Here's how the part is built. I have some questions about the finished solid (model axes, mm). A direction names the side the tool comes from. Coordinates: 2 decimals unless noted, no trailing zeros. Order: outer loops, then holes, each group sorted by start corner. A loop starts at its lowest first (then second) coordinate and runs counter-clockwise, first axis right, second up. Notation, with made-up numbers: M 15.5,56 L 24.5,56 A25 cw 24.5,75 Z; hole C -15.5,7.5 d2. An arc over 180 degrees is marked long. Answer as CSV lines item,"result". Start each with the question number.
Autodesk Inventor part; units mm, degrees
ref_plane "Start plane" through (0, 0, 0) normal (0, 0, 1) x (1, 0, 0)
ref_plane "End plane" through (0, 0, 1323.975) normal (0, 0, 1) x (1, 0, 0)
ref_plane "YZ Plane" through (0, 0, 0) normal (1, 0, 0) x (0, 1, 0)
ref_plane "Start plane" through (0, 0, 0) normal (0, 0, 1) x (1, 0, 0)
ref_plane "End plane" through (0, 0, 1323.975) normal (0, 0, 1) x (1, 0, 0)
sketch "Sketch" plane through (0, 0, 0) normal (0, 0, 1) x (1, 0, 0)
  line L0 (0, 76.2) -> (0, 0)
  line L1 (0, 0) -> (50.8, 0)
  line L2 (50.8, 0) -> (50.8, 2.7625)
  line L3 (48.8, 4.7625) -> (12.6365, 4.7625)
  line L4 (4.7625, 12.6365) -> (4.7625, 74.2)
  line L5 (2.7625, 76.2) -> (0, 76.2)
  line L6 (-7.0414, 0) -> (21.5385, 0) construction
  line L7 (0, -8.0414) -> (0, 34.5385) construction
  arc A0 (4.7625, 12.6365) -> (12.6365, 4.7625) centre (12.6365, 12.6365) ccw
  arc A1 (50.8, 2.7625) -> (48.8, 4.7625) centre (48.8, 2.7625) ccw
  arc A2 (4.7625, 74.2) -> (2.7625, 76.2) centre (2.7625, 74.2) ccw
  line L8 (0, 93.5453) -> (0, -24.9725) construction
  line L9 (-18.6925, 0) -> (62.8653, 0) construction
  point P0 (50.8, 4.7625)
  point P1 (4.7625, 4.7625)
  point P2 (4.7625, 76.2)
  dimension "d12" = 4.7625
  dimension "d13" = 76.2
  dimension "d14" = 50.8
  dimension "d15" = 0
  dimension "d16" = 4.7625
  dimension "d17" = 0
  dimension "d18" = 7.874
  dimension "d19" = 2
extrude "Body" add sketch "Sketch" along normal up to surface (1323.975 mm away) from surface at 0
equation "\"d12\" = G_T"
equation "\"d13\" = G_H"
equation "\"d14\" = G_W"
equation "\"d16\" = G_T"
equation "\"d18\" = G_IR"
equation "\"d4\" = G_L"
equation "\"G_W\" = 50.8"
equation "\"G_H\" = 76.2"
equation "\"G_T\" = 4.7625"
equation "\"G_ER\" = 4.064"
equation "\"G_IR\" = 7.874"
equation "\"G_L\" = B_L + G_OFFSET_START + G_OFFSET_END"
equation "\"ex\" = 0"
equation "\"ey\" = 0"
equation "\"G_OFFSET_START\" = 0"
equation "\"G_OFFSET_END\" = 0"
equation "\"d21\" = G_OFFSET_END + B_L"
equation "\"B_L\" = 1323.975"
properties part number "ANSI L 3 x 2 x 3_16 00000008"
1) Suppose I cut it at B-B on y = 61.5. Please give me the cut outline in (x, z) (1 decimal), plus the area to 3 significant figures.
2) I need wall thicknesses on line 1 (Y direction, x = 43.5, z = 872.5); line 2 (Y direction, x = 4, z = 751). Which ranges of each line are inside material? Lowest first, please. Write a range as [from, to].
3) Will these pins go through, and if not, where does the flat tip stop? pin 1 Ø5 at (x, z) = (36.5, 988) entering from -Y; pin 2 Ø18 at (x, z) = (24.5, 622.5) entering from +Y; pin 3 Ø6 at (y, z) = (27.5, 880.5) entering from +X.
4) Suppose I cut it at A-A on z = 379. Please give me the cut outline in (x, y).
5) Which directions (+Z, -Z, +X, -X, +Y, -Y) give clear straight access to the entire face, cutting with the end or side of a thin tool? Please do faces 1 (the face through (0, 39, 653)), 2 (the face through (31, 4.762, 653)).
Output:
1,outline,"M 0,0 L 4.8,0 L 4.8,1324 L 0,1324 Z"
1,area,"6,310 mm²"
2,line 1,"[0, 4.76]"
2,line 2,"[0, 75.77]"
3,pin 1,"y = 0"
3,pin 2,"y = 4.76"
3,pin 3,"x = 4.76"
4,outline,"M 0,0 L 50.8,0 L 50.8,2.76 A2 ccw 48.8,4.76 L 12.64,4.76 A7.87 cw 4.76,12.64 L 4.76,74.2 A2 ccw 2.76,76.2 L 0,76.2 Z"
5,face 1,"+Z, -Z, -X, +Y, -Y"
5,face 2,"+Z, -Z, +X, +Y"
